from build123d import *

# Parameters (mm, degrees)
SKETCH1_W               = 60
SKETCH1_H               = 72
BOTTOM_DEPTH            = 2
SKETCH2_R               = 2.25
PIN_LOCS_DEPTH          = 4
SKETCH5_R               = 1.25
PIN_HOLES_DEPTH         = 4
SKETCH3_R               = 2.25
SKETCH3_R_2             = 2.15
SENSOR_PINS_DEPTH       = 8
SKETCH6_R               = 1.25
SKETCH6_R_2             = 1.2
PIN_HOLES_SENSORS_DEPTH = 4
SKETCH4_W               = 8
SKETCH4_H               = 10
POWER_CABLE_DEPTH       = 2
SKETCH7_W               = 16.5
SKETCH7_H               = 25
SKETCH7_W_2             = 17
SKETCH7_H_2             = 13
SKETCH7_W_3             = 15.833991833
SKETCH7_W_4             = 13.166008167
SKETCH7_W_5             = 15.5
CUT_EXTRUDE1_DEPTH      = 2
SKETCH8_W               = 64.981954188
SKETCH8_H               = 18.550894708
CUT_EXTRUDE2_DEPTH      = 30
SKETCH9_W               = 66.656683173
SKETCH9_H               = 21.371664799
CUT_EXTRUDE3_DEPTH      = 10
SKETCH10_W              = 36.941564119
SKETCH10_H              = 17.072061012
CUT_EXTRUDE4_DEPTH      = 10
SKETCH12_W              = 38.10862574
SKETCH12_H              = 18.099687976
CUT_EXTRUDE5_DEPTH      = 3
SKETCH13_W              = 10
SKETCH13_H              = 2
BOSS_EXTRUDE1_DEPTH     = 17
SKETCH14_W              = 11.076631965
SKETCH14_H              = 2
BOSS_EXTRUDE2_DEPTH     = 8


with BuildPart() as part:
    # Sketch1 → Bottom (new body)
    with BuildSketch(Plane(origin=(0, 0, 0), x_dir=(1, 0, 0), z_dir=(0, 1, 0))):
        Rectangle(SKETCH1_W, SKETCH1_H)
    extrude(amount=BOTTOM_DEPTH)

    # Sketch2 → Pin Locs (add)
    with BuildSketch(Plane(origin=(0, 2, 0), x_dir=(1, 0, 0), z_dir=(0, 1, 0))):
        with Locations(Location((25.7, -13.1, 0), (0, 0, 90))):
            Circle(SKETCH2_R)
        with Locations(Location((-20.7, -13.1, 0), (0, 0, 270))):
            Circle(SKETCH2_R)
        with Locations(Location((25.7, -31.5, 0), (0, 0, 270))):
            Circle(SKETCH2_R)
        with Locations(Location((-20.7, -31.5, 0), (0, 0, 90))):
            Circle(SKETCH2_R)
    extrude(amount=PIN_LOCS_DEPTH)

    # Sketch5 → Pin Holes (cut)
    with BuildSketch(Plane(origin=(0, 6, 0), x_dir=(1, 0, 0), z_dir=(0, 1, 0))):
        with Locations(Location((-20.7, -31.5, 0), (0, 0, 270))):
            Circle(SKETCH5_R)
        with Locations(Location((-20.7, -13.1, 0), (0, 0, 270))):
            Circle(SKETCH5_R)
        with Locations(Location((25.7, -13.1, 0), (0, 0, 270))):
            Circle(SKETCH5_R)
        with Locations(Location((25.7, -31.5, 0), (0, 0, 270))):
            Circle(SKETCH5_R)
    extrude(amount=-PIN_HOLES_DEPTH, mode=Mode.SUBTRACT)

    # Sketch3 → Sensor Pins (add)
    with BuildSketch(Plane(origin=(0, 2, 0), x_dir=(1, 0, 0), z_dir=(0, 1, 0))):
        with Locations(Location((20.7, 19.7, 0), (0, 0, 270))):
            Circle(SKETCH3_R)
        with Locations(Location((20.7, -1.2, 0), (0, 0, 90))):
            Circle(SKETCH3_R)
        with Locations(Location((7.5, -1.2, 0), (0, 0, 270))):
            Circle(SKETCH3_R)
        with Locations(Location((7.5, 19.7, 0), (0, 0, 90))):
            Circle(SKETCH3_R)
        with Locations(Location((-1.1, 19.7, 0), (0, 0, 270))):
            Circle(SKETCH3_R_2)
        with Locations(Location((-1.1, -1.2, 0), (0, 0, 90))):
            Circle(SKETCH3_R_2)
        with Locations(Location((-14.3, -1.2, 0), (0, 0, 270))):
            Circle(SKETCH3_R_2)
        with Locations(Location((-14.3, 19.7, 0), (0, 0, 90))):
            Circle(SKETCH3_R_2)
    extrude(amount=SENSOR_PINS_DEPTH)

    # Sketch6 → Pin Holes Sensors (cut)
    with BuildSketch(Plane(origin=(0, 10, 0), x_dir=(1, 0, 0), z_dir=(0, 1, 0))):
        with Locations(Location((-14.3, -1.2, 0), (0, 0, 270))):
            Circle(SKETCH6_R)
        with Locations(Location((-1.1, -1.2, 0), (0, 0, 270))):
            Circle(SKETCH6_R)
        with Locations(Location((-1.1, 19.7, 0), (0, 0, 270))):
            Circle(SKETCH6_R_2)
        with Locations(Location((-14.3, 19.7, 0), (0, 0, 270))):
            Circle(SKETCH6_R_2)
        with Locations(Location((20.7, -1.2, 0), (0, 0, 270))):
            Circle(SKETCH6_R_2)
        with Locations(Location((20.7, 19.7, 0), (0, 0, 270))):
            Circle(SKETCH6_R_2)
        with Locations(Location((7.5, 19.7, 0), (0, 0, 270))):
            Circle(SKETCH6_R_2)
        with Locations(Location((7.5, -1.2, 0), (0, 0, 270))):
            Circle(SKETCH6_R_2)
    extrude(amount=-PIN_HOLES_SENSORS_DEPTH, mode=Mode.SUBTRACT)

    # Sketch4 → Power Cable (cut)
    with BuildSketch(Plane(origin=(0, 2, 0), x_dir=(1, 0, 0), z_dir=(0, 1, 0))):
        with Locations((26, 31)):
            Rectangle(SKETCH4_W, SKETCH4_H)
    extrude(amount=-POWER_CABLE_DEPTH, mode=Mode.SUBTRACT)

    # Sketch7 → Cut-Extrude1 (cut)
    with BuildSketch(Plane(origin=(0, 2, 0), x_dir=(1, 0, 0), z_dir=(0, 1, 0))):
        with Locations((-7.75, -20.5)):
            Rectangle(SKETCH7_W, SKETCH7_H)
        with Locations((-18.5, 9.5)):
            Rectangle(SKETCH7_W_2, SKETCH7_H_2)
        with Locations((1.916995917, 9.5)):
            Rectangle(SKETCH7_W_3, SKETCH7_H_2)
        with Locations((20.416995916, 9.5)):
            Rectangle(SKETCH7_W_4, SKETCH7_H_2)
        with Locations((12.25, -20.5)):
            Rectangle(SKETCH7_W_5, SKETCH7_H)
    extrude(amount=-CUT_EXTRUDE1_DEPTH, mode=Mode.SUBTRACT)

    # Sketch8 → Cut-Extrude2 (cut)
    with BuildSketch(Plane.XY.offset(36)):
        with Locations((-0.087810816, 5.992805319)):
            Rectangle(SKETCH8_W, SKETCH8_H)
    extrude(amount=-CUT_EXTRUDE2_DEPTH, mode=Mode.SUBTRACT)

    # Sketch9 → Cut-Extrude3 (cut)
    with BuildSketch(Plane(origin=(0, 0, -36), x_dir=(-1, 0, 0), z_dir=(0, 0, -1))):
        with Locations((-0.680170236, 4.633119296)):
            Rectangle(SKETCH9_W, SKETCH9_H)
    extrude(amount=-CUT_EXTRUDE3_DEPTH, mode=Mode.SUBTRACT)

    # Sketch10 → Cut-Extrude4 (cut)
    with BuildSketch(Plane.ZY.offset(30)):
        with Locations((-9.291501149, 5.008650235)):
            Rectangle(SKETCH10_W, SKETCH10_H)
    extrude(amount=-CUT_EXTRUDE4_DEPTH, mode=Mode.SUBTRACT)

    # Sketch12 → Cut-Extrude5 (cut)
    with BuildSketch(Plane(origin=(30, 0, 0), x_dir=(0, 0, -1), z_dir=(1, 0, 0))):
        with Locations((8.949912617, 4.668826375)):
            Rectangle(SKETCH12_W, SKETCH12_H)
    extrude(amount=-CUT_EXTRUDE5_DEPTH, mode=Mode.SUBTRACT)

    # Sketch13 → Boss-Extrude1 (add)
    with BuildSketch(Plane(origin=(0, 0, -26), x_dir=(-1, 0, 0), z_dir=(0, 0, -1))):
        with Locations((15, 1)):
            Rectangle(SKETCH13_W, SKETCH13_H)
    extrude(amount=BOSS_EXTRUDE1_DEPTH)

    # Sketch14 → Boss-Extrude2 (add)
    with BuildSketch(Plane.XY.offset(6)):
        with Locations((4.13094739, 1)):
            Rectangle(SKETCH14_W, SKETCH14_H)
    extrude(amount=BOSS_EXTRUDE2_DEPTH)


solid = part.part
Read the model definition and answer for the solid it produces. Units are mm, in the model's axes. A direction names the side the tool comes from. Give positions to 0.01 mm unless a question says otherwise; leave off trailing zeros. Write each loop counter-clockwise with the first axis right and the second up, starting at its lowest first coordinate (ties: lowest second). Pieces come first, ordered by that corner, then holes. Notation, with made-up numbers: (81, 9) - (104, 9) arc R19 cw to (104, 18) - close; hole circle Ø8 at (18.5, -10). An arc over 180 degrees is marked (long way). Answer in a Markdown table with one row per item. Add a question column.
Item 1: A tool of negligible diameter and unlimited length cuts with its end or side. For faces 1 (the face through (20, 1, -16)), 2 (the face through (8, 6, -20)), 3 (the face through (2, 1, -16)), from which of +Z, -Z, +X, -X, +Y, -Y can it reach the whole face along a straight path? Write none if from no direction.
Item 2: Determine the mould class of faces 4 (the face through (-16.11, 5.94, -20.86)), 5 (the face through (-10, 1, -9)), 6 (the face through (8, 6, 1)), 7 (the face through (8, 10, -21)) for opening direction X: pulls with the +X half, pulls with the -X half, needs draft (parallel to the pull), parting line crosses it, or undercut.
Item 3: Flat-ended cylindrical pins translate along their axes: P1, Ø1.2, axis at x = 20.5, z = -20, coming from the +Y side; P2, Ø1, axis at y = 1, z = -8.5, coming from the -X side; P3, Ø1.6, axis at y = 1, z = -9.5, coming from the +X side. Find the tip coordinate at first contact, or state that the pin passes through.
Item 4: Find the intervals of material crossed by L1, parallel to X at y = 3.5, z = -18.5; L2, parallel to Y at x = 16, z = 4.5; L3, parallel to Z at x = 24.5, y = 1, in increasing order.
Item 5: Section D-D, the plane x = 7.5 is taken. Write down the section's boundary in (y, z), and give its area (3 significant figures).
Item 6: Section C-C, the plane z = -11.5 is taken. Write down the section's boundary in (x, y), and give its area (3 significant figures).
Item 7: Section B-B, the plane y = 9 is taken. Count the separate pieces of the cut face and the enclosed holes in it, and give its area (3 significant figures).
Item 8: Section A-A, the plane x = 20.7 is taken. Write down the section's boundary in (y, z), and give its area (3 significant figures).
Recorded:
| question | item | result |
|---|---|---|
| 1 | face 1 | +X, +Y, -Y |
| 1 | face 2 | +Y |
| 1 | face 3 | +Y, -Y |
| 2 | face 4 | undercut |
| 2 | face 5 | pulls with the -X half |
| 2 | face 6 | undercut |
| 2 | face 7 | needs draft |
| 3 | P1 | stops at y = 6 |
| 3 | P2 | stops at x = -10 |
| 3 | P3 | stops at x = 13.83 |
| 4 | L1 | x = -16.08 to -12.52, -2.88 to 0.68, 5.6 to 9.4, 18.8 to 22.6 |
| 4 | L2 | y = 0 to 2 |
| 4 | L3 | z = -26 to -16, -3 to 6 |
| 5 | outline | (0, -26) - (2, -26) - (2, -21.95) - (10, -21.95) - (10, -20.9) - (6, -20.9) - (6, -18.5) - (10, -18.5) - (10, -17.45) - (2, -17.45) - (2, -16) - (0, -16) - close; (0, -3) - (2, -3) - (2, -1.05) - (10, -1.05) - (10, 0) - (6, 0) - (6, 2.4) - (10, 2.4) - (10, 3.45) - (2, 3.45) - (2, 14) - (0, 14) - close |
| 5 | area | 107 mm2 |
| 6 | outline | (-10, 0) - (-6, 0) - (-6, 2) - (-10, 2) - close; (9.83, 0) - (13.83, 0) - (13.83, 2) - (9.83, 2) - close |
| 6 | area | 16.0 mm2 |
| 7 | separate pieces | 8 |
| 7 | enclosed holes | 8 |
| 7 | area | 84.7 mm2 |
| 8 | outline | (0, -26) - (2, -26) - (2, -21.95) - (10, -21.95) - (10, -20.9) - (6, -20.9) - (6, -18.5) - (10, -18.5) - (10, -17.45) - (2, -17.45) - (2, -16) - (0, -16) - close; (0, -3) - (2, -3) - (2, -1.05) - (10, -1.05) - (10, 0) - (6, 0) - (6, 2.4) - (10, 2.4) - (10, 3.45) - (2, 3.45) - (2, 6) - (0, 6) - close |
| 8 | area | 90.8 mm2 |
